```python
from build123d import *

# Parameters (mm, degrees)
SKETCH1_W                = 400
SKETCH1_H                = 3
BASE_FLANGE1_DEPTH       = 290
CUT_EXTRUDE1_REACH       = 354.291
EDGE_FLANGE1_START       = -6
EDGE_FLANGE1_DEPTH       = 7
EDGE_FLANGE1_START_2     = -0.31686
EDGE_FLANGE1_2_OUTLINE_W = 3
EDGE_FLANGE1_2_OUTLINE_H = 80
EDGE_FLANGE1_2_DEPTH     = 1.31686
EDGE_FLANGE1_START_3     = -50
EDGE_FLANGE1_3_OUTLINE_W = 3
EDGE_FLANGE1_3_OUTLINE_H = 80
EDGE_FLANGE1_3_DEPTH     = 44
EDGE_FLANGE1_START_4     = 110
EDGE_FLANGE1_4_DEPTH     = 80
EDGE_FLANGE1_5_DEPTH     = 80
SKETCH15_R               = 2.5
CUT_EXTRUDE2_DEPTH       = 497.588360717
FILLET1_R                = 7
SKETCH16_R               = 2.5
CUT_EXTRUDE3_DEPTH       = 10
CUT_EXTRUDE4_REACH       = 357.4
SKETCH17_R               = 2.5
CUT_EXTRUDE5_REACH       = 357.809


with BuildPart() as part:
    # Base-Flange1: sheet metal written as solids
    # Sketch1 → Base-Flange1 (new body)
    with BuildSketch(Plane.XY):
        with Locations((0, -1.5)):
            Rectangle(SKETCH1_W, SKETCH1_H)
    extrude(amount=BASE_FLANGE1_DEPTH)

    # Sketch6 → Cut-Extrude1 (cut, up to next)
    with BuildSketch(Plane.XZ.offset(3), mode=Mode.PRIVATE) as cut_extrude1_sk1:
        Polygon((200, 0), (150, 50), (-150, 50), (-200, 0), align=None)
    cut_extrude1_tool1 = extrude(cut_extrude1_sk1.sketch, amount=-CUT_EXTRUDE1_REACH, mode=Mode.PRIVATE) & part.part
    add(cut_extrude1_tool1.solids().sort_by_distance((0, -3, 23.809524))[0], mode=Mode.SUBTRACT)

    # Edge-Flange1: read off the stored shape, not the designer's step
    # Edge-Flange1 outline → Edge-Flange1 (cut)
    with BuildSketch(Plane(origin=(0, 0, 0), x_dir=(1, 0, 0), z_dir=(0, 1, 0)).offset(EDGE_FLANGE1_START)):
        with BuildLine():
            Line((200, -193), (200, -190))
            Line((200, -190), (191, -190))
            ThreePointArc((191, -190), (189.5, -191.5), (191, -193))
            Line((191, -193), (200, -193))
        make_face()
        with BuildLine():
            Line((191, -110), (200, -110))
            Line((200, -110), (200, -107))
            Line((200, -107), (191, -107))
            ThreePointArc((191, -107), (189.5, -108.5), (191, -110))
        make_face()
        with BuildLine():
            Line((-200, -107), (-200, -110))
            Line((-200, -110), (-191, -110))
            ThreePointArc((-191, -110), (-189.5, -108.5), (-191, -107))
            Line((-191, -107), (-200, -107))
        make_face()
        with BuildLine():
            Line((-191, -190), (-200, -190))
            Line((-200, -190), (-200, -193))
            Line((-200, -193), (-191, -193))
            ThreePointArc((-191, -193), (-189.5, -191.5), (-191, -190))
        make_face()
    extrude(amount=EDGE_FLANGE1_DEPTH, mode=Mode.SUBTRACT)

    # Edge-Flange1 2 outline → Edge-Flange1 2 (cut)
    with BuildSketch(Plane(origin=(0, 0, 0), x_dir=(1, 0, 0), z_dir=(0, 1, 0)).offset(EDGE_FLANGE1_START_2)):
        with Locations((198.5, -150)):
            Rectangle(EDGE_FLANGE1_2_OUTLINE_W, EDGE_FLANGE1_2_OUTLINE_H)
        with Locations((-198.5, -150)):
            Rectangle(EDGE_FLANGE1_2_OUTLINE_W, EDGE_FLANGE1_2_OUTLINE_H)
    extrude(amount=EDGE_FLANGE1_2_DEPTH, mode=Mode.SUBTRACT)

    # Edge-Flange1 4 outline → Edge-Flange1 4 (cut)
    with BuildSketch(Plane.XY.offset(EDGE_FLANGE1_START_4)):
        with BuildLine():
            Line((-200, -3), (-199.196152423, -3))
            ThreePointArc((-199.196152423, -3), (-197, -0.803847577), (-194, 0))
            Line((-194, 0), (-197, 0))
            Line((-197, 0), (-197, -0.31686))
            Line((-197, -0.31686), (-200, -0.31686))
            Line((-200, -0.31686), (-200, -3))
        make_face()
        with BuildLine():
            Line((197, 0), (194, 0))
            ThreePointArc((194, 0), (197, -0.803847577), (199.196152423, -3))
            Line((199.196152423, -3), (200, -3))
            Line((200, -3), (200, -0.31686))
            Line((200, -0.31686), (197, -0.31686))
            Line((197, -0.31686), (197, 0))
        make_face()
    extrude(amount=EDGE_FLANGE1_4_DEPTH, mode=Mode.SUBTRACT)



with BuildPart() as body_2:
    # Edge-Flange1 3 outline → Edge-Flange1 3 (new body)
    with BuildSketch(Plane(origin=(0, 0, 0), x_dir=(1, 0, 0), z_dir=(0, 1, 0)).offset(EDGE_FLANGE1_START_3)):
        with Locations((198.5, -150)):
            Rectangle(EDGE_FLANGE1_3_OUTLINE_W, EDGE_FLANGE1_3_OUTLINE_H)
        with Locations((-198.5, -150)):
            Rectangle(EDGE_FLANGE1_3_OUTLINE_W, EDGE_FLANGE1_3_OUTLINE_H)
    extrude(amount=EDGE_FLANGE1_3_DEPTH)


with BuildPart() as part_1:
    add(part.part)

    add(body_2.part)  # Edge-Flange1 5 merges body 2
    # Edge-Flange1 5 outline → Edge-Flange1 5 (add)
    with BuildSketch(Plane.XY.offset(EDGE_FLANGE1_START_4)):
        with BuildLine():
            ThreePointArc((-199.196152423, -3), (-199.795554958, -4.447085729), (-200, -6))
            Line((-200, -6), (-197, -6))
            ThreePointArc((-197, -6), (-196.121320344, -3.878679656), (-194, -3))
            Line((-194, -3), (-199.196152423, -3))
        make_face()
        with BuildLine():
            Line((199.196152423, -3), (194, -3))
            ThreePointArc((194, -3), (196.121320344, -3.878679656), (197, -6))
            Line((197, -6), (200, -6))
            ThreePointArc((200, -6), (199.795554958, -4.447085729), (199.196152423, -3))
        make_face()
    extrude(amount=EDGE_FLANGE1_5_DEPTH)

    # Sketch15 → Cut-Extrude2 (cut, through all)
    with BuildSketch(Plane(origin=(200, 0, 0), x_dir=(0, 0, -1), z_dir=(1, 0, 0))):
        with Locations(Location((-165, -28, 0), (0, 0, 90))):
            Circle(SKETCH15_R)
        with Locations(Location((-135, -17, 0), (0, 0, 90))):
            Circle(SKETCH15_R)
        with Locations(Location((-135, -39, 0), (0, 0, 90))):
            Circle(SKETCH15_R)
    extrude(amount=-CUT_EXTRUDE2_DEPTH, mode=Mode.SUBTRACT)

    # Fillet1
    fillet1_edges = [part_1.edges().sort_by_distance(p)[0] for p in [
        (-150, -1.5, 50),
        (150, -1.5, 50),
        (-200, -1.5, 0),
        (200, -1.5, 0),
    ]]
    fillet(fillet1_edges, radius=FILLET1_R)

    # Sketch16 → Cut-Extrude3 (cut)
    with BuildSketch(Plane(origin=(0, 0, 0), x_dir=(1, 0, 0), z_dir=(0, 1, 0))):
        with Locations(Location((0, -60, 0), (0, 0, 270))):
            Circle(SKETCH16_R)
        with Locations(Location((80, -60, 0), (0, 0, 270))):
            Circle(SKETCH16_R)
        with Locations(Location((-80, -60, 0), (0, 0, 90))):
            Circle(SKETCH16_R)
    extrude(amount=-CUT_EXTRUDE3_DEPTH, mode=Mode.SUBTRACT)

    # Sketch17 → Cut-Extrude4 (cut, up to next)
    with BuildSketch(Plane.XZ.offset(3), mode=Mode.PRIVATE) as cut_extrude4_sk1:
        with Locations(Location((-125, 279.5, 0), (0, 0, 270))):
            Circle(SKETCH17_R)
    cut_extrude4_tool1 = extrude(cut_extrude4_sk1.sketch, amount=-CUT_EXTRUDE4_REACH, mode=Mode.PRIVATE) & part_1.part
    # Sketch17 → Cut-Extrude4 (cut, up to next)
    with BuildSketch(Plane.XZ.offset(3), mode=Mode.PRIVATE) as cut_extrude4_sk2:
        with Locations(Location((-125, 100.5, 0), (0, 0, 270))):
            Circle(SKETCH17_R)
    cut_extrude4_tool2 = extrude(cut_extrude4_sk2.sketch, amount=-CUT_EXTRUDE4_REACH, mode=Mode.PRIVATE) & part_1.part
    # Sketch17 → Cut-Extrude4 (cut, up to next)
    with BuildSketch(Plane.XZ.offset(3), mode=Mode.PRIVATE) as cut_extrude4_sk3:
        with Locations(Location((-75, 279.5, 0), (0, 0, 270))):
            Circle(SKETCH17_R)
    cut_extrude4_tool3 = extrude(cut_extrude4_sk3.sketch, amount=-CUT_EXTRUDE4_REACH, mode=Mode.PRIVATE) & part_1.part
    # Sketch17 → Cut-Extrude4 (cut, up to next)
    with BuildSketch(Plane.XZ.offset(3), mode=Mode.PRIVATE) as cut_extrude4_sk4:
        with Locations(Location((-75, 100.5, 0), (0, 0, 270))):
            Circle(SKETCH17_R)
    cut_extrude4_tool4 = extrude(cut_extrude4_sk4.sketch, amount=-CUT_EXTRUDE4_REACH, mode=Mode.PRIVATE) & part_1.part
    # Sketch17 → Cut-Extrude4 (cut, up to next)
    with BuildSketch(Plane.XZ.offset(3), mode=Mode.PRIVATE) as cut_extrude4_sk5:
        with Locations(Location((-25, 279.5, 0), (0, 0, 270))):
            Circle(SKETCH17_R)
    cut_extrude4_tool5 = extrude(cut_extrude4_sk5.sketch, amount=-CUT_EXTRUDE4_REACH, mode=Mode.PRIVATE) & part_1.part
    # Sketch17 → Cut-Extrude4 (cut, up to next)
    with BuildSketch(Plane.XZ.offset(3), mode=Mode.PRIVATE) as cut_extrude4_sk6:
        with Locations(Location((-25, 100.5, 0), (0, 0, 270))):
            Circle(SKETCH17_R)
    cut_extrude4_tool6 = extrude(cut_extrude4_sk6.sketch, amount=-CUT_EXTRUDE4_REACH, mode=Mode.PRIVATE) & part_1.part
    # Sketch17 → Cut-Extrude4 (cut, up to next)
    with BuildSketch(Plane.XZ.offset(3), mode=Mode.PRIVATE) as cut_extrude4_sk7:
        with Locations(Location((25, 279.5, 0), (0, 0, 270))):
            Circle(SKETCH17_R)
    cut_extrude4_tool7 = extrude(cut_extrude4_sk7.sketch, amount=-CUT_EXTRUDE4_REACH, mode=Mode.PRIVATE) & part_1.part
    # Sketch17 → Cut-Extrude4 (cut, up to next)
    with BuildSketch(Plane.XZ.offset(3), mode=Mode.PRIVATE) as cut_extrude4_sk8:
        with Locations(Location((25, 100.5, 0), (0, 0, 270))):
            Circle(SKETCH17_R)
    cut_extrude4_tool8 = extrude(cut_extrude4_sk8.sketch, amount=-CUT_EXTRUDE4_REACH, mode=Mode.PRIVATE) & part_1.part
    # Sketch17 → Cut-Extrude4 (cut, up to next)
    with BuildSketch(Plane.XZ.offset(3), mode=Mode.PRIVATE) as cut_extrude4_sk9:
        with Locations(Location((75, 279.5, 0), (0, 0, 270))):
            Circle(SKETCH17_R)
    cut_extrude4_tool9 = extrude(cut_extrude4_sk9.sketch, amount=-CUT_EXTRUDE4_REACH, mode=Mode.PRIVATE) & part_1.part
    # Sketch17 → Cut-Extrude4 (cut, up to next)
    with BuildSketch(Plane.XZ.offset(3), mode=Mode.PRIVATE) as cut_extrude4_sk10:
        with Locations(Location((75, 100.5, 0), (0, 0, 270))):
            Circle(SKETCH17_R)
    cut_extrude4_tool10 = extrude(cut_extrude4_sk10.sketch, amount=-CUT_EXTRUDE4_REACH, mode=Mode.PRIVATE) & part_1.part
    # Sketch17 → Cut-Extrude4 (cut, up to next)
    with BuildSketch(Plane.XZ.offset(3), mode=Mode.PRIVATE) as cut_extrude4_sk11:
        with Locations(Location((125, 279.5, 0), (0, 0, 270))):
            Circle(SKETCH17_R)
    cut_extrude4_tool11 = extrude(cut_extrude4_sk11.sketch, amount=-CUT_EXTRUDE4_REACH, mode=Mode.PRIVATE) & part_1.part
    # Sketch17 → Cut-Extrude4 (cut, up to next)
    with BuildSketch(Plane.XZ.offset(3), mode=Mode.PRIVATE) as cut_extrude4_sk12:
        with Locations(Location((125, 100.5, 0), (0, 0, 270))):
            Circle(SKETCH17_R)
    cut_extrude4_tool12 = extrude(cut_extrude4_sk12.sketch, amount=-CUT_EXTRUDE4_REACH, mode=Mode.PRIVATE) & part_1.part
    add(cut_extrude4_tool1.solids().sort_by_distance((-125, -3, 279.5))[0], mode=Mode.SUBTRACT)
    add(cut_extrude4_tool2.solids().sort_by_distance((-125, -3, 100.5))[0], mode=Mode.SUBTRACT)
    add(cut_extrude4_tool3.solids().sort_by_distance((-75, -3, 279.5))[0], mode=Mode.SUBTRACT)
    add(cut_extrude4_tool4.solids().sort_by_distance((-75, -3, 100.5))[0], mode=Mode.SUBTRACT)
    add(cut_extrude4_tool5.solids().sort_by_distance((-25, -3, 279.5))[0], mode=Mode.SUBTRACT)
    add(cut_extrude4_tool6.solids().sort_by_distance((-25, -3, 100.5))[0], mode=Mode.SUBTRACT)
    add(cut_extrude4_tool7.solids().sort_by_distance((25, -3, 279.5))[0], mode=Mode.SUBTRACT)
    add(cut_extrude4_tool8.solids().sort_by_distance((25, -3, 100.5))[0], mode=Mode.SUBTRACT)
    add(cut_extrude4_tool9.solids().sort_by_distance((75, -3, 279.5))[0], mode=Mode.SUBTRACT)
    add(cut_extrude4_tool10.solids().sort_by_distance((75, -3, 100.5))[0], mode=Mode.SUBTRACT)
    add(cut_extrude4_tool11.solids().sort_by_distance((125, -3, 279.5))[0], mode=Mode.SUBTRACT)
    add(cut_extrude4_tool12.solids().sort_by_distance((125, -3, 100.5))[0], mode=Mode.SUBTRACT)

    # Sketch18 → Cut-Extrude5 (cut, up to next)
    with BuildSketch(Plane(origin=(0, 0, 0), x_dir=(1, 0, 0), z_dir=(0, 1, 0)), mode=Mode.PRIVATE) as cut_extrude5_sk1:
        with BuildLine():
            Line((50, -200), (-50, -200))
            ThreePointArc((-50, -200), (-60, -190), (-50, -180))
            Line((-50, -180), (50, -180))
            ThreePointArc((50, -180), (60, -190), (50, -200))
        make_face()
    cut_extrude5_tool1 = extrude(cut_extrude5_sk1.sketch, amount=-CUT_EXTRUDE5_REACH, mode=Mode.PRIVATE) & part_1.part
    add(cut_extrude5_tool1.solids().sort_by_distance((0, 0, 190))[0], mode=Mode.SUBTRACT)


solid = part_1.part
```
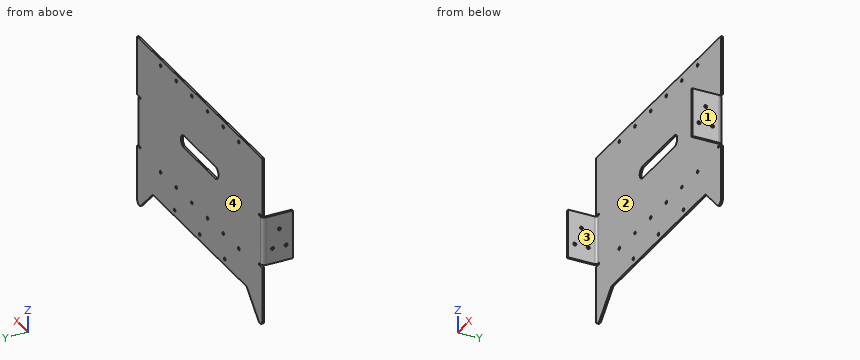
Geometry check sheet. Reference: the model listing, model coordinates, mm. Face numbers are marked on the shaded views. Give positions to 0.01 mm unless a question says otherwise; leave off trailing zeros. Order: outer loops, then holes, each group sorted by start corner. A loop starts at its lowest first (then second) coordinate and runs counter-clockwise, first axis right, second up. Notation, with made-up numbers: (21.5, 6) -> (46.5, 6) arc R21 ccw to (46.5, 40) -> close; hole circle Ø3 at (33.25, 46.25). An arc over 180 degrees is marked (long way). Write each question's results on one line, items separated by ' | '. Start each with the question number.
(1) Mould release check, pull along X, two halves, no side actions. Record for the marked faces 1, 2, 3 and 4: pulls with the +X half, pulls with the -X half, needs draft (parallel to the pull), parting line crosses it, or undercut.
(2) Sectioned sample at A-A (x = -164.5). Enter the section's corners in (y, z).
(3) Gauge pin test, flat ends, axial feed: P1, Ø6.5, axis at x = 125, z = 279.5, coming from the -Y side; P2, Ø6, axis at x = -25, z = 279.5, coming from the +Y side; P3, Ø0.9, axis at x = 2.5, y = -2, coming from the -Z side; P4, Ø10, axis at x = -197.5, y = -27.5, coming from the -Z side. Record the tip position at first contact, or that the pin passes through.
(4) Scan lines: line 1 (X direction, y = -0.65, z = 60); line 2 (Z direction, x = 198.9, y = -28); line 3 (X direction, y = -37, z = 138). Record each from-to range of solid material in increasing order.
(5) Sectioned sample at B-B (z = 248). Enter the section's corners in (x, y), plus the area to 3 significant figures.
Answer below:
1) face 1: pulls with the +X half | face 2: undercut | face 3: undercut | face 4: needs draft
2) outline: (-3, 35.5) -> (0, 35.5) -> (0, 290) -> (-3, 290) -> close
3) P1: y = -3 | P2: y = 0 | P3: z = 50 | P4: z = 110
4) line 1: -200 to -82.5, -77.5 to -2.5, 2.5 to 77.5, 82.5 to 200 | line 2: 110 to 162.5, 167.5 to 190 | line 3: -200 to -197, 197 to 200
5) outline: (-200, -3) -> (200, -3) -> (200, 0) -> (-200, 0) -> close | area: 1,200 mm2
